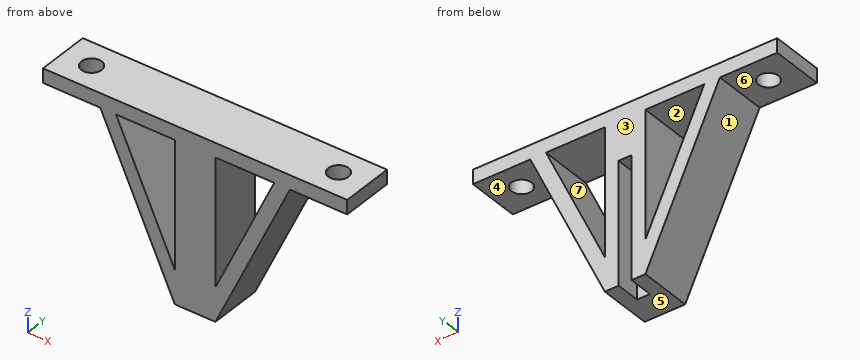
from build123d import *

# Parameters (mm, degrees)
SKETCH1_W           = 3.2
SKETCH1_H           = 13
BOSS_EXTRUDE1_DEPTH = 13
SKETCH1_6_W         = 3.2
SKETCH1_6_H         = 30
BOSS_EXTRUDE2_DEPTH = 7
SKETCH2_R           = 2.5
CUT_EXTRUDE1_DEPTH  = 7


with BuildPart() as part:
    # Sketch1 → Boss-Extrude1 (new body)
    with BuildSketch(Plane(origin=(0, 0, 0), x_dir=(1, 0, 0), z_dir=(0, 1, 0))):
        Polygon((-20.111109043, -23.976958525), (-5.599078341, 7.223907484), (-5.599078341, 15.523041475), (-23.971171364, -23.976958525), align=None)
        Polygon((-25.599078341, -27.476958525), (-5.599078341, -27.476958525), (-5.599078341, -23.976958525), (-20.111109043, -23.976958525), (-23.971171364, -23.976958525), (-38.099078341, -23.976958525), (-38.099078341, -27.476958525), align=None)
        Polygon((-5.599078341, -23.976958525), (-5.599078341, -27.476958525), (-2.199078341, -27.476958525), (-2.199078341, -14.476958525), (-2.199078341, 15.523041475), (-5.599078341, 15.523041475), (-5.599078341, 7.223907484), align=None)
        Polygon((1.000921659, -14.476958525), (1.000921659, -27.476958525), (4.400921659, -27.476958525), (4.400921659, -23.976958525), (4.400921659, 7.223907484), (4.400921659, 15.523041475), (1.000921659, 15.523041475), align=None)
        with Locations((-0.599078341, -20.976958525)):
            Rectangle(SKETCH1_W, SKETCH1_H)
        Polygon((4.400921659, -23.976958525), (4.400921659, -27.476958525), (24.400921659, -27.476958525), (36.900921659, -27.476958525), (36.900921659, -23.976958525), (22.773014682, -23.976958525), (4.400921659, 15.523041475), (4.400921659, 7.223907484), (18.912952361, -23.976958525), align=None)
    extrude(amount=BOSS_EXTRUDE1_DEPTH)

    # Sketch1_6 → Boss-Extrude2 (add)
    with BuildSketch(Plane(origin=(0, 0, 0), x_dir=(1, 0, 0), z_dir=(0, 1, 0))):
        with Locations((-0.599078341, 0.523041475)):
            Rectangle(SKETCH1_6_W, SKETCH1_6_H)
    extrude(amount=BOSS_EXTRUDE2_DEPTH)

    # Sketch2 → Cut-Extrude1 (cut)
    with BuildSketch(Plane(origin=(0, 0, 23.976958525), x_dir=(-1, 0, 0), z_dir=(0, 0, -1))):
        with Locations((31.035124853, 6.5)):
            Circle(SKETCH2_R)
        with Locations((-29.836968171, 6.5)):
            Circle(SKETCH2_R)
    extrude(amount=-CUT_EXTRUDE1_DEPTH, mode=Mode.SUBTRACT)


solid = part.part
Here's how the part is built. I have some questions about the finished solid (model axes, mm). Face numbers are marked on the shaded views. A direction names the side the tool comes from. Coordinates: 2 decimals unless noted, no trailing zeros. Order: outer loops, then holes, each group sorted by start corner. A loop starts at its lowest first (then second) coordinate and runs counter-clockwise, first axis right, second up. Notation, with made-up numbers: (-1.75, 4) -> (55.25, 4) arc R29 ccw to (55.25, 31) -> close; hole circle Ø2 at (-12, 36.5). An arc over 180 degrees is marked (long way). Answer in a Markdown table with one row per item.
(1) I want a section at C-C on z = 10. List the corners of the cut face in (x, y) for me.
Answer key:
| item | result |
|---|---|
| outline | (-17.47, 0) -> (-13.61, 0) -> (-13.61, 13) -> (-17.47, 13) -> close; (-5.6, 0) -> (4.4, 0) -> (4.4, 13) -> (1, 13) -> (1, 7) -> (-2.2, 7) -> (-2.2, 13) -> (-5.6, 13) -> close; (12.41, 0) -> (16.27, 0) -> (16.27, 13) -> (12.41, 13) -> close |
(2) I want a section at B-B on x = 5.5. List the corners of the cut face in (y, z) for me.
Answer key:
| item | result |
|---|---|
| outline | (0, -13.16) -> (13, -13.16) -> (13, -4.86) -> (0, -4.86) -> close; (0, 23.98) -> (13, 23.98) -> (13, 27.48) -> (0, 27.48) -> close |
(3) I want a section at D-D on x = 24.5. List the corners of the cut face in (y, z) for me.
Answer key:
| item | result |
|---|---|
| outline | (0, 23.98) -> (13, 23.98) -> (13, 27.48) -> (0, 27.48) -> close |
(4) Please list where these lines run through material, in increasing order: probe 1 along X at (y, z) = (0.75, -5.5); probe 2 along X at (y, z) = (2.5, 16.5); probe 3 along Z at (x, y) = (-19.5, 5).
Answer key:
| item | result |
|---|---|
| probe 1 | -10.26 to -6.4, -5.6 to 4.4, 5.2 to 9.06 |
| probe 2 | -20.49 to -16.63, -5.6 to 4.4, 15.44 to 19.3 |
| probe 3 | 14.36 to 22.66, 23.98 to 27.48 |
(5) Will these pins go through, and if not, where does the flat tip stop? pin 1 Ø4 at (x, y) = (-15, 9) entering from -Z; pin 2 Ø6.5 at (x, y) = (29.84, 6.5) entering from -Z; pin 3 Ø1.8 at (y, z) = (9, 2) entering from -X; pin 4 Ø2.5 at (x, z) = (-1, 1.5) entering from +Y.
Answer key:
| item | result |
|---|---|
| pin 1 | z = 0.39 |
| pin 2 | z = 23.98 |
| pin 3 | x = -14.17 |
| pin 4 | y = 13 |
(6) On a 3-axis mill with a long thin cutter (end or side, diameter ignored), from which of +Z, -Z, +X, -X, +Y, -Y can I reach the whole of each face in a straight line? I mean the marked faces 4, 5, 6 and 7. Say none if no direction works.
Answer key:
| item | result |
|---|---|
| face 4 | -Z, +X, +Y, -Y |
| face 5 | -Z, +X, -X, +Y, -Y |
| face 6 | -Z, -X, +Y, -Y |
| face 7 | +Y, -Y |
(7) I want a section at A-A on y = 11.75. List the corners of the cut face in (x, z) for me.
Answer key:
| item | result |
|---|---|
| outline | (-38.1, 23.98) -> (-23.97, 23.98) -> (-5.6, -15.52) -> (-2.2, -15.52) -> (-2.2, 14.48) -> (1, 14.48) -> (1, -15.52) -> (4.4, -15.52) -> (22.77, 23.98) -> (36.9, 23.98) -> (36.9, 27.48) -> (-38.1, 27.48) -> close; hole (-20.11, 23.98) -> (-5.6, -7.22) -> (-5.6, 23.98) -> close; hole (4.4, -7.22) -> (18.91, 23.98) -> (4.4, 23.98) -> close |
(8) Thinking about a two-plate mould opening in Z: for the marked faces 1, 2 and 3, which applies, +Z half, -Z half, draft (parallel to the pull), parting line (faces both ways), or undercut?
Answer key:
| item | result |
|---|---|
| face 1 | -Z half |
| face 2 | undercut |
| face 3 | draft |
